Design review of the part built by this model. Coordinates are the model's own, in mm. Face numbers are marked on the shaded views. Coordinates: 2 decimals unless noted, no trailing zeros. Write each loop counter-clockwise with the first axis right and the second up, starting at its lowest first coordinate (ties: lowest second). Pieces come first, ordered by that corner, then holes. Notation, with made-up numbers: (-25.5, 52.5) -> (22.5, 52.5) arc R10 cw to (22.5, 62.5) -> close; hole circle Ø7 at (20, 11.5). An arc over 180 degrees is marked (long way). Answer in a Markdown table with one row per item. Add a question column.
Item 1: Clearance check with flat-ended pins moving along their axes: P1, Ø6, axis at x = 23.75, y = 18.125, coming from the -Z side (3 decimals); P2, Ø4, axis at x = 33, y = 8, coming from the -Z side; P3, Ø5, axis at x = -71.25, y = 18.125, coming from the -Z side; P4, Ø8.5, axis at x = 73, y = -3.5, coming from the +Z side. State where each tip first meets the part, or that it passes through.
Item 2: Take a section at D-D, the plane x = -5. Write out the cut boundary in (y, z) (3 decimals), and give its area (3 significant figures).
Item 3: Draft analysis for pull direction Y (two halves, no side actions). For the marked faces 1, 2 and 3, state which applies: released by +Y, released by -Y, zero draft, split by the parting line, or undercut.
Item 4: Take a section at B-B, the plane x = 43. Write out the cut boundary in (y, z) (3 decimals), and give its area (3 significant figures).
Item 5: To check wall thickness, follow line 1 (Y direction, x = 23.75, z = 10.25) (3 decimals); line 2 (Y direction, x = 30.5, z = 7.25) (3 decimals); line 3 (X direction, y = 18, z = 7.5). State the ranges of each line that lie inside material, in increasing order.
Item 6: Take a section at A-A, the plane x = 71.25. Write out the cut boundary in (y, z) (3 decimals).
Item 7: Take a section at C-C, the plane y = -0.5. Write out the cut boundary in (x, z), and give its area (3 significant figures).
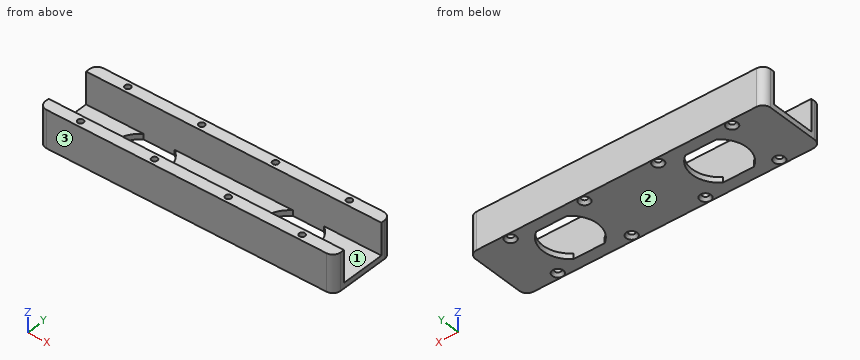
from build123d import *

# Parameters (mm, degrees)
BOSS_EXTRUDE4_DEPTH                            = 3.5
SKETCH6_W                                      = 190
SKETCH6_H                                      = 7.5
BOSS_EXTRUDE5_DEPTH                            = 20.5
CSK_FOR_6_FLAT_HEAD_MACHINE_SCREW1_D           = 3.7973
CSK_FOR_6_FLAT_HEAD_MACHINE_SCREW1_CSINK_D     = 7.0866
CSK_FOR_6_FLAT_HEAD_MACHINE_SCREW1_CSINK_ANGLE = 82
FILLET1_R                                      = 5


with BuildPart() as part:
    # Sketch5 → Boss-Extrude4 (new body)
    with BuildSketch(Plane.XY):
        Polygon((95, 21.875), (95, 14.375), (95, -14.375), (95, -21.875), (-95, -21.875), (-95, -14.375), (-95, 14.375), (-95, 21.875), align=None)
        with BuildLine():
            Line((57.980449639, 14.375), (38.019550361, 14.375))
            ThreePointArc((38.019550361, 14.375), (30.5, 0), (38.019550361, -14.375))
            Line((38.019550361, -14.375), (57.980449639, -14.375))
            ThreePointArc((57.980449639, -14.375), (65.5, 0), (57.980449639, 14.375))
        make_face(mode=Mode.SUBTRACT)
        with BuildLine():
            Line((-57.980449639, -14.375), (-38.019550361, -14.375))
            ThreePointArc((-38.019550361, -14.375), (-30.5, 0), (-38.019550361, 14.375))
            Line((-38.019550361, 14.375), (-57.980449639, 14.375))
            ThreePointArc((-57.980449639, 14.375), (-65.5, 0), (-57.980449639, -14.375))
        make_face(mode=Mode.SUBTRACT)
    extrude(amount=BOSS_EXTRUDE4_DEPTH)

    # Sketch6 → Boss-Extrude5 (add)
    with BuildSketch(Plane.XY.offset(3.5)):
        with Locations((0, 18.125)):
            Rectangle(SKETCH6_W, SKETCH6_H)
        with Locations((0, -18.125)):
            Rectangle(SKETCH6_W, SKETCH6_H)
    extrude(amount=BOSS_EXTRUDE5_DEPTH)

    # CSK for #6 Flat Head Machine Screw1 (through all)
    with Locations(Plane(origin=(0, 0, 0), x_dir=(-1, 0, 0), z_dir=(0, 0, -1))):
        with Locations((71.25, 18.125), (23.75, 18.125), (-23.75, 18.125), (-71.25, 18.125), (71.25, -18.125), (23.75, -18.125), (-23.75, -18.125), (-71.25, -18.125)):
            CounterSinkHole(CSK_FOR_6_FLAT_HEAD_MACHINE_SCREW1_D / 2, CSK_FOR_6_FLAT_HEAD_MACHINE_SCREW1_CSINK_D / 2, counter_sink_angle=CSK_FOR_6_FLAT_HEAD_MACHINE_SCREW1_CSINK_ANGLE)

    # Fillet1
    fillet1_edges = [part.edges().sort_by_distance(p)[0] for p in [
        (95, 21.875, 12),
        (95, -21.875, 12),
        (-95, -21.875, 12),
        (-95, 21.875, 12),
    ]]
    fillet(fillet1_edges, radius=FILLET1_R)


solid = part.part
Answers:
| question | item | result |
|---|---|---|
| 1 | P1 | stops at z = 0.625 |
| 1 | P2 | stops at z = 0 |
| 1 | P3 | stops at z = 1.2 |
| 1 | P4 | stops at z = 3.5 |
| 2 | outline | (-21.875, 0) -> (21.875, 0) -> (21.875, 24) -> (14.375, 24) -> (14.375, 3.5) -> (-14.375, 3.5) -> (-14.375, 24) -> (-21.875, 24) -> close |
| 2 | area | 461 mm^2 |
| 3 | face 1 | undercut |
| 3 | face 2 | zero draft |
| 3 | face 3 | released by -Y |
| 4 | outline | (-21.875, 0) -> (-14.375, 0) -> (-14.375, 24) -> (-21.875, 24) -> close; (14.375, 0) -> (21.875, 0) -> (21.875, 24) -> (14.375, 24) -> close |
| 4 | area | 360 mm^2 |
| 5 | line 1 | y = -21.875 to -20.024, -16.226 to -14.375, 14.375 to 16.226, 20.024 to 21.875 |
| 5 | line 2 | y = -21.875 to -14.375, 14.375 to 21.875 |
| 5 | line 3 | x = -94.87 to -73.14, -69.36 to -25.64, -21.86 to 21.86, 25.64 to 69.36, 73.14 to 94.87 |
| 6 | outline | (-21.875, 0) -> (-21.668, 0) -> (-20.024, 1.892) -> (-20.024, 24) -> (-21.875, 24) -> close; (-16.226, 1.892) -> (-14.582, 0) -> (14.582, 0) -> (16.226, 1.892) -> (16.226, 24) -> (14.375, 24) -> (14.375, 3.5) -> (-14.375, 3.5) -> (-14.375, 24) -> (-16.226, 24) -> close; (20.024, 1.892) -> (21.668, 0) -> (21.875, 0) -> (21.875, 24) -> (20.024, 24) -> close |
| 7 | outline | (-95, 0) -> (-65.49, 0) -> (-65.49, 3.5) -> (-95, 3.5) -> close; (-30.51, 0) -> (30.51, 0) -> (30.51, 3.5) -> (-30.51, 3.5) -> close; (65.49, 0) -> (95, 0) -> (95, 3.5) -> (65.49, 3.5) -> close |
| 7 | area | 420 mm^2 |
